Model file for the job. Use its own axes, mm. Coordinates: 2 decimals unless noted, no trailing zeros. Order: outer loops, then holes, each group sorted by start corner. A loop starts at its lowest first (then second) coordinate and runs counter-clockwise, first axis right, second up. Notation, with made-up numbers: (8, 83) -> (19, 83) arc R28 ccw to (19, 121) -> close; hole circle Ø3 at (9, -10.75). An arc over 180 degrees is marked (long way). Write item = value, one per line. Start each with the question number.
Q1. Cut at A-A, the plane y = -2.75. List the corners of the cut face in (x, z).
Q2. Flat gauge pins, fed straight in: pin 1 (4 mm diameter, centred on y = -0.5, z = -3, fed in from +X); pin 2 (1.5 mm diameter, centred on y = -1.5, z = -1.5, fed in from -X); pin 3 (1.7 mm diameter, centred on x = -0.5, z = -1, fed in from -Y); pin 4 (5 mm diameter, centred on x = -1, y = -1.5, fed in from +Z). Where does each tip first touch, or does it go through?
Q3. Cut at B-B, the plane y = -8.75. List the corners of the cut face in (x, z).
Q4. Wall check: line 1 (X direction, y = 0.75, z = 4). Give the ranges that are in metal, low to high. Write a range as from..to.
from build123d import *

# Parameters (mm, degrees)
SKETCH1_R           = 5.1
SKETCH1_R_2         = 5
SKETCH8_R           = 5.1
BOSS_EXTRUDE2_DEPTH = 0.1
SKETCH9_R           = 4
BOSS_EXTRUDE3_DEPTH = 8
SKETCH10_R          = 3.95
CUT_EXTRUDE1_DEPTH  = 11.84573649
SKETCH12_4_R        = 3
SKETCH12_4_R_2      = 2.9
EXTRUDE_THIN2_DEPTH = 1


# Read off the part's stored shape, not the designer's step: Loft-Thin7
with BuildPart() as part:
    # Sweep-Thin1: sweep along a path in Sketch3
    with BuildLine(Plane(origin=(0, 0, 0), x_dir=(0, 0, -1), z_dir=(1, 0, 0))) as sweep_thin1_path:
        Line((0, 0), (0, 1))
    # Sketch1 → Sweep-Thin1 (sweep)
    with BuildSketch(Plane(origin=(0, 0, 0), x_dir=(1, 0, 0), z_dir=(0, 1, 0))):
        Circle(SKETCH1_R)
        Circle(SKETCH1_R_2, mode=Mode.SUBTRACT)
    sweep(path=sweep_thin1_path.line)

    # Sketch8 → Boss-Extrude2 (add)
    with BuildSketch(Plane(origin=(0, 0, 0), x_dir=(-1, 0, 0), z_dir=(0, -1, 0))):
        with Locations(Location((0, 0, 0), (0, 0, 270))):
            Circle(SKETCH8_R)
    extrude(amount=BOSS_EXTRUDE2_DEPTH)

    # Sketch9 → Boss-Extrude3 (add)
    with BuildSketch(Plane(origin=(0, -0.1, 0), x_dir=(-1, 0, 0), z_dir=(0, -1, 0))):
        with Locations(Location((0, 0, 0), (0, 0, 90))):
            Circle(SKETCH9_R)
    extrude(amount=BOSS_EXTRUDE3_DEPTH)

    # Sketch10 → Cut-Extrude1 (cut, through all)
    with BuildSketch(Plane(origin=(0, 0, 0), x_dir=(1, 0, 0), z_dir=(0, 1, 0))):
        with Locations(Location((0, 0, 0), (0, 0, 270))):
            Circle(SKETCH10_R)
    extrude(amount=-CUT_EXTRUDE1_DEPTH, mode=Mode.SUBTRACT)

    # Loft-Thin7 outline → Loft-Thin7 (revolve)
    with BuildSketch(Plane.XY):
        Polygon((4, -8.1), (3.776393202, -8.1), (2.776393202, -8.6), (3, -8.6), align=None)
    revolve(axis=Axis((0, 0, 0), (0, 1, 0)))

    # Sketch12<4> → Extrude-Thin2 (add)
    with BuildSketch(Plane(origin=(0, -8.6, 0), x_dir=(-1, 0, 0), z_dir=(0, -1, 0))):
        Circle(SKETCH12_4_R)
        Circle(SKETCH12_4_R_2, mode=Mode.SUBTRACT)
    extrude(amount=EXTRUDE_THIN2_DEPTH)

    # Sketch16 → Revolve-Thin2 (revolve)
    with BuildSketch(Plane.XY, mode=Mode.PRIVATE) as revolve_thin2_sk:
        Polygon((0, -9.6), (0, -10.1), (3, -9.6), align=None)
        Polygon((0.1, -9.7), (0.1, -9.981953958), (1.791723747, -9.7), align=None, mode=Mode.SUBTRACT)
    revolve(revolve_thin2_sk.sketch.rotate(Axis((0, -16.369174854, 0), (0, 1, 0)), 270), axis=Axis((0, -16.369174854, 0), (0, 1, 0)))


solid = part.part
Here are the results:
q1.outline = circle Ø8 at (0, 0); hole circle Ø7.9 at (0, 0)
q2.pin_1 = 4.99
q2.pin_2 = -3.93
q2.pin_3 = -10.06
q2.pin_4 = 5.1
q3.outline = circle Ø6 at (0, 0); hole circle Ø5.8 at (0, 0)
q4.line_1 = -3.16..-3, 3..3.16
